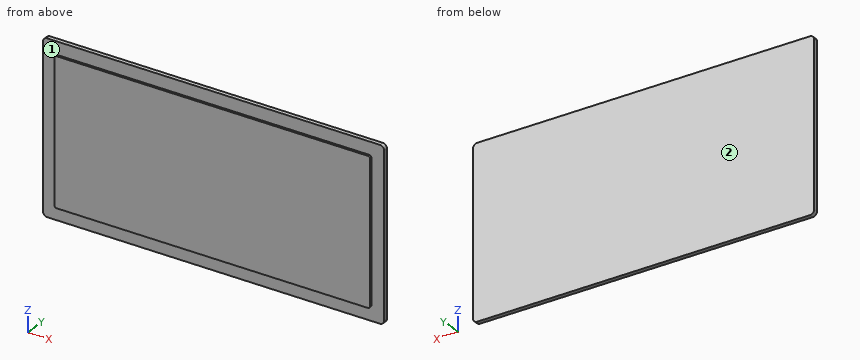
from build123d import *

# Parameters (mm, degrees)
F0_W     = 80
F0_H     = 40
F1_DEPTH = 1
F2_W     = 74
F2_H     = 34
F3_DEPTH = 0.5
F4_R     = 1
F5_R     = 0.5


with BuildPart() as f1:
    # F0 (on Front) → F1 (new body)
    with BuildSketch(Plane.XZ):
        Rectangle(F0_W, F0_H)
    extrude(amount=F1_DEPTH)

    # F2 (on face) → F3 (join)
    with BuildSketch(Plane.XZ.offset(1)):
        Rectangle(F2_W, F2_H)
    extrude(amount=F3_DEPTH)

    # F4
    f4_edges = [f1.edges().sort_by_distance(p)[0] for p in [
        (40, -0.5, 20),
        (40, -0.5, -20),
        (-40, -0.5, -20),
        (-40, -0.5, 20),
    ]]
    fillet(f4_edges, radius=F4_R)

    # F5
    f5_edges = [f1.edges().sort_by_distance(p)[0] for p in [
        (-37, -1.25, 17),
        (-37, -1.25, -17),
        (37, -1.25, -17),
        (37, -1.25, 17),
    ]]
    fillet(f5_edges, radius=F5_R)


solid = f1.part
CAD build for the part. Positions are in the model's coordinates, mm. Face numbers are marked on the shaded views. A direction names the side the tool comes from. Coordinates: 2 decimals unless noted, no trailing zeros. Loops run counter-clockwise (first coordinate to the right, second up) from the corner with the lowest first, then second, coordinate; pieces in that order, holes last. Notation, with made-up numbers: (59.25, -14) - (69.25, -14) arc R21 ccw to (69.25, 4) - close; hole circle Ø2 at (-0.5, -30). An arc over 180 degrees is marked (long way). Write item = value, one per line. Start each with the question number.
Q1. Drill centre line: L1, parallel to Z at x = -13, y = -1.05. Where is it in solid material? Low to high.
Q2. Cut at B-B, the plane x = -31. List the corners of the cut face in (y, z), then the cut area to 3 significant figures.
Q3. Which spindle directions (+Z, -Z, +X, -X, +Y, -Y) get a long thin tool onto all of the face, cutting with end or side? Do the marked faces 1 and 2. Say none if no direction does.
Q4. Cut at A-A, the plane z = -10.5. List the corners of the cut face in (x, y), then the cut area to 3 significant figures.
Q5. Flat gauge pin, fed straight in: pin 1 Ø0.6 at (x, y) = (-8.5, -1.5) entering from -Z. Where does the tip first touch, or does it go through?
Computed:
q1.L1 = -17 to 17
q2.outline = (-1.5, -17) - (-1, -17) - (-1, -20) - (0, -20) - (0, 20) - (-1, 20) - (-1, 17) - (-1.5, 17) - close
q2.area = 57.0 mm²
q3.face_1 = -Y
q3.face_2 = +Z, -Z, +X, -X, +Y
q4.outline = (-40, -1) - (-37, -1) - (-37, -1.5) - (37, -1.5) - (37, -1) - (40, -1) - (40, 0) - (-40, 0) - close
q4.area = 117 mm²
q5.pin_1 = -17
